Geometry check sheet. Reference: the model listing, model coordinates, mm. Face numbers are marked on the shaded views. A direction names the side the tool comes from. Round coordinates to 2 decimals unless told otherwise and drop trailing zeros. Order: outer loops, then holes, each group sorted by start corner. A loop starts at its lowest first (then second) coordinate and runs counter-clockwise, first axis right, second up. Notation, with made-up numbers: (-20.75, -24) -> (-16.75, -24) arc R20 ccw to (-16.75, -9) -> close; hole circle Ø3 at (-20.5, -17.5). An arc over 180 degrees is marked (long way). Use a Markdown table: item, result. Add a question column.
Item 1: Gauge pin test, flat ends, axial feed: pin 1 Ø17 at (y, z) = (-1, 30.5) entering from +X; pin 2 Ø2 at (x, z) = (-19, 27.5) entering from +Y; pin 3 Ø2 at (x, z) = (-44, 21) entering from -Y. Record the tip position at first contact, or that the pin passes through.
Item 2: Sectioned sample at C-C, the plane z = 43. Record the cut outline in (x, y).
Item 3: Set-up check for the marked faces 1, 2, 3, 4 and 5: record each of +Z, -Z, +X, -X, +Y, -Y from which the full face is reachable in a straight line by a thin tool's end or side.
Item 4: Sectioned sample at B-B, the plane x = -43. Record the cut outline in (y, z).
Item 5: Sectioned sample at A-A, the plane y = 0. Record the cut outline in (x, z).
Item 6: Material ranges on probe 1 along Z at (x, y) = (6.5, -28.5); probe 2 along Z at (x, y) = (-2.5, 15); probe 3 along X at (y, z) = (12, 29), recorded low to high. Write a range as [from, to].
Item 7: Sectioned sample at D-D, the plane z = 22. Record the cut outline in (x, y).
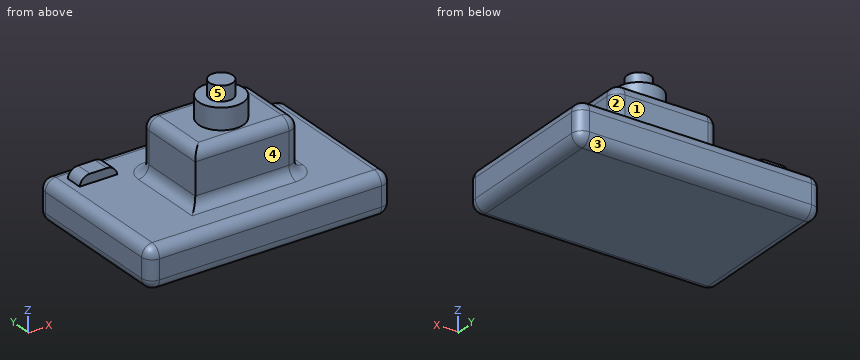
from build123d import *

# Parameters (mm, degrees)
F0_W        = 116.8206892908
F0_H        = 76.6635760665
F1_DEPTH    = 19.558
F2_R        = 5.08
F3_W        = 50.0696562231
F3_H        = 37.0959769934
F4_DEPTH    = 25.4
F5_F1_R     = 5.08
F5_F2_R     = 5.08
F6_W        = 18.107265234
F6_H        = 8.2995928824
F7_DEPTH    = 4.318
F8_T1_DEPTH = 33.4122171977
F9_R        = 10.7094586845
F10_DEPTH   = 10.16
F11_R       = 5.6111694278
F12_DEPTH   = 7.112


# Not quite as in the source:
# - a fillet or chamfer that OpenCascade refuses, or shapes differently, is made with other operations: its cross-section is extruded or revolved along the edge and cut away or added


with BuildPart() as f1:
    # F0 (on Top) → F1 (new body)
    with BuildSketch(Plane.XY):
        with Locations((-1.5465151519, 2.0281374454)):
            Rectangle(F0_W, F0_H)
    extrude(amount=F1_DEPTH)

    # F2
    f2_edges = [f1.edges().sort_by_distance(p)[0] for p in [
        (56.863829, 2.028137, 19.558),
        (-1.546515, 40.359925, 19.558),
        (-59.95686, 2.028137, 19.558),
        (-1.546515, -36.303651, 19.558),
        (-1.546515, -36.303651, 0),
        (56.863829, 2.028137, 0),
        (-1.546515, 40.359925, 0),
        (-59.95686, 2.028137, 0),
        (-59.95686, 40.359925, 9.779),
        (-59.95686, -36.303651, 9.779),
        (56.863829, 40.359925, 9.779),
        (56.863829, -36.303651, 9.779),
    ]]
    fillet(f2_edges, radius=F2_R)

    # F3 (on face) → F4 (join)
    with BuildSketch(Plane.XY.offset(19.558)):
        with Locations((0.8830688894, 1.7247768119)):
            Rectangle(F3_W, F3_H)
    extrude(amount=F4_DEPTH)

    # F5: fillet of radius 5.08 on 10 edges, made by hand

    # F5_f1
    f5_f1_edges = [f1.edges().sort_by_distance(p)[0] for p in [
        (0.8830688894, -16.8232116848, 44.958),
        (-24.1517592221, 1.7247768119, 44.958),
        (0.8830688894, 20.2727653086, 44.958),
        (25.9178970009, 1.7247768119, 44.958),
        (25.9178970009, -16.8232116848, 32.258),
        (25.9178970009, 20.2727653086, 32.258),
        (-24.1517592221, 20.2727653086, 32.258),
    ]]
    fillet(f5_f1_edges, radius=F5_F1_R)

    # F5_f2
    f5_f2_edges = [f1.edges().sort_by_distance(p)[0] for p in [
        (25.9178970009, 1.7247768119, 19.558),
        (-24.1517592221, -0.8152231881, 19.558),
        (0.8830688894, 20.2727653086, 19.558),
        (24.4299994493, 18.784867757, 19.558),
        (-22.6638616706, 18.784867757, 19.558),
        (24.4299994493, -15.3353141333, 19.558),
    ]]
    fillet(f5_f2_edges, radius=F5_F2_R)

    # F6 (on face) → F7 (join)
    with BuildSketch(Plane.XY.offset(19.558)):
        with Locations((-42.6498092711, 27.5764670223)):
            Rectangle(F6_W, F6_H)
    extrude(amount=F7_DEPTH)

    # F8: fillet of radius 5.08 on 2 edges, made by hand

    # F8_s2 → F8_t1 (cut)
    with BuildSketch(Plane.XZ.offset(-44.2825756211)):
        with BuildLine():
            ThreePointArc((-51.7034418881, 19.558), (-49.9926718469, 22.6481007256), (-46.680917025, 23.876))
            Line((-46.680917025, 23.876), (-51.7034418881, 23.876))
            Line((-51.7034418881, 23.876), (-51.7034418881, 19.558))
        make_face()
        with BuildLine():
            ThreePointArc((-33.5961766541, 19.558), (-35.3069466953, 22.6481007256), (-38.6187015172, 23.876))
            Line((-38.6187015172, 23.876), (-33.5961766541, 23.876))
            Line((-33.5961766541, 23.876), (-33.5961766541, 19.558))
        make_face()
    extrude(amount=F8_T1_DEPTH, mode=Mode.SUBTRACT)

    # F9 (on face) → F10 (join)
    with BuildSketch(Plane.XY.offset(44.958)):
        Circle(F9_R)
    extrude(amount=F10_DEPTH)

    # F11 (on face) → F12 (join)
    with BuildSketch(Plane.XY.offset(55.118)):
        Circle(F11_R)
    extrude(amount=F12_DEPTH)


solid = f1.part
Found:
| question | item | result |
|---|---|---|
| 1 | pin 1 | stops at x = 26.66 |
| 1 | pin 2 | stops at y = 20.27 |
| 1 | pin 3 | stops at y = 23.43 |
| 2 | outline | (-23.08, -15.75) -> (20.84, -15.75) arc R4.01 ccw to (24.85, -11.74) -> (24.85, 15.19) arc R4.01 ccw to (20.84, 19.2) -> (-19.07, 19.2) arc R4.01 ccw to (-23.08, 15.19) -> close |
| 3 | face 1 | +Z, +X, -X, +Y |
| 3 | face 2 | +Z, +X, +Y |
| 3 | face 3 | -Z, +X, -X, +Y |
| 3 | face 4 | +Z, +X, -X, -Y |
| 3 | face 5 | +Z |
| 4 | outline | (-36.3, 5.08) arc R5.08 ccw to (-31.22, 0) -> (35.28, 0) arc R5.08 ccw to (40.36, 5.08) -> (40.36, 14.48) arc R5.08 ccw to (35.28, 19.56) -> (31.73, 19.56) -> (31.73, 23.88) -> (23.43, 23.88) -> (23.43, 19.56) -> (-31.22, 19.56) arc R5.08 ccw to (-36.3, 14.48) -> close |
| 5 | outline | (-59.96, 5.08) arc R5.08 ccw to (-54.88, 0) -> (51.78, 0) arc R5.08 ccw to (56.86, 5.08) -> (56.86, 14.48) arc R5.08 ccw to (51.78, 19.56) -> (31, 19.56) arc R5.08 cw to (25.92, 24.64) -> (25.92, 39.88) arc R5.08 ccw to (20.84, 44.96) -> (10.71, 44.96) -> (10.71, 55.12) -> (5.61, 55.12) -> (5.61, 62.23) -> (-5.61, 62.23) -> (-5.61, 55.12) -> (-10.71, 55.12) -> (-10.71, 44.96) -> (-19.07, 44.96) arc R5.08 ccw to (-24.15, 39.88) -> (-24.15, 24.64) arc R5.08 cw to (-29.23, 19.56) -> (-54.88, 19.56) arc R5.08 ccw to (-59.96, 14.48) -> close |
| 6 | probe 1 | z = [0, 19.56] |
| 6 | probe 2 | z = [0, 44.96] |
| 6 | probe 3 | x = [-24.15, 25.92] |
| 7 | outline | (-50.62, 23.43) -> (-34.68, 23.43) -> (-34.68, 31.73) -> (-50.62, 31.73) -> close; (-24.89, -17.56) -> (20.84, -17.56) arc R5.82 ccw to (26.66, -11.74) -> (26.66, 15.19) arc R5.82 ccw to (20.84, 21.01) -> (-19.07, 21.01) arc R5.82 ccw to (-24.89, 15.19) -> close |
